CAD build for the part. Positions are in the model's coordinates, mm. A direction names the side the tool comes from. Coordinates: 2 decimals unless noted, no trailing zeros. Write each loop counter-clockwise with the first axis right and the second up, starting at its lowest first coordinate (ties: lowest second). Pieces come first, ordered by that corner, then holes. Notation, with made-up numbers: (45, -32) - (83, -32) arc R8 cw to (83, -17) - close; hole circle Ø1 at (47, -10.5). An arc over 180 degrees is marked (long way). Answer in a Markdown table with one row per item. Add a question column.
Q1. Band-saw the part on B-B (x = 0). List the corners of the cut face in (y, z).
Q2. Two-plate mould, pull along Y, no slides. Class faces 1 (the flat face through (3, -5, 115.824)), 2 (the cylindrical face through (-4.434, -3.4, 120.582)), 3 (the flat face through (0, 0, 11.176)), 4 (the cylindrical face through (0.06, 0.09, -4.32)): +Y half, -Y half, draft (parallel to the pull), parting line (faces both ways), or undercut.
Q3. 3-axis set-ups, long thin cutter, end or side, ignore diameter. For faces 5 (the flat face through (-3.937, 0, -4)), 6 (the flat face through (0, -5.588, -6)), 7 (the cylindrical face through (-1.915, -1.468, 69.126)), 8 (the flat face through (0, 5.588, -6)), 9 (the flat face through (3.937, 0, -4)): which of +Z, -Z, +X, -X, +Y, -Y reach the whole face in a straight line?
Q4. Drill centre lines: line 1 along Y through (x, z) = (0, 51); line 2 along X through (y, z) = (0.25, 56); line 3 along Y through (x, z) = (-1.5, -6.35). Where is each one in solid material? Low to high. Write a range as from..to.
Q5. Pin check, flat tips, straight feed: pin 1 (3.5 mm diameter, centred on y = 1, z = -5, fed in from -X); pin 2 (4 mm diameter, centred on x = 1, z = -3.5, fed in from -Y); pin 3 (4 mm diameter, centred on x = -1, y = 1, fed in from +Z); pin 4 (2.5 mm diameter, centred on x = 0, y = 1, fed in from +Z). Stop position of each tip, or through.
Q6. Band-saw the part on A-A (y = 0). List the corners of the cut face in (x, z), and give its area (3 significant figures).
Q7. Band-saw the part on D-D (z = 106). List the corners of the cut face in (x, y), and give its area (3 significant figures).
Q8. Band-saw the part on C-C (z = -6.35). List the corners of the cut face in (x, y).
```python
from build123d import *

# Parameters (mm, degrees)
SKETCH1_R           = 7.874
BOSS_EXTRUDE1_DEPTH = 115.824
SKETCH2_R           = 5.588
BOSS_EXTRUDE2_DEPTH = 9.652
SKETCH3_W           = 7.874
SKETCH3_H           = 11.176
BOSS_EXTRUDE3_DEPTH = 11.176
SKETCH4_R           = 2.032
CUT_EXTRUDE1_DEPTH  = 12.811
SKETCH5_R           = 2.413
CUT_EXTRUDE2_DEPTH  = 114.3


with BuildPart() as part:
    # Sketch1 → Boss-Extrude1 (new body)
    with BuildSketch(Plane.XY):
        Circle(SKETCH1_R)
    extrude(amount=BOSS_EXTRUDE1_DEPTH)

    # Sketch2 → Boss-Extrude2 (add)
    with BuildSketch(Plane.XY.offset(115.824)):
        Circle(SKETCH2_R)
    extrude(amount=BOSS_EXTRUDE2_DEPTH)

    # Sketch3 → Boss-Extrude3 (add)
    with BuildSketch(Plane(origin=(0, 0, 0), x_dir=(-1, 0, 0), z_dir=(0, 0, -1))):
        Rectangle(SKETCH3_W, SKETCH3_H)
    extrude(amount=BOSS_EXTRUDE3_DEPTH)

    # Sketch4 → Cut-Extrude1 (cut, through all)
    with BuildSketch(Plane(origin=(3.937, 0, 0), x_dir=(0, 0, -1), z_dir=(1, 0, 0))):
        with Locations((6.35, 0)):
            Circle(SKETCH4_R)
    extrude(amount=-CUT_EXTRUDE1_DEPTH, mode=Mode.SUBTRACT)

    # Sketch5 → Cut-Extrude2 (cut)
    with BuildSketch(Plane.XY.offset(125.476)):
        Circle(SKETCH5_R)
    extrude(amount=-CUT_EXTRUDE2_DEPTH, mode=Mode.SUBTRACT)


solid = part.part
```
Checked values:
| question | item | result |
|---|---|---|
| 1 | outline | (-7.87, 0) - (-5.59, 0) - (-5.59, -11.18) - (5.59, -11.18) - (5.59, 0) - (7.87, 0) - (7.87, 115.82) - (5.59, 115.82) - (5.59, 125.48) - (2.41, 125.48) - (2.41, 11.18) - (-2.41, 11.18) - (-2.41, 125.48) - (-5.59, 125.48) - (-5.59, 115.82) - (-7.87, 115.82) - close; hole circle Ø4.06 at (0, -6.35) |
| 2 | face 1 | draft |
| 2 | face 2 | parting line |
| 2 | face 3 | undercut |
| 2 | face 4 | undercut |
| 3 | face 5 | -Z, -X, +Y, -Y |
| 3 | face 6 | -Z, +X, -X, -Y |
| 3 | face 7 | +Z |
| 3 | face 8 | -Z, +X, -X, +Y |
| 3 | face 9 | -Z, +X, +Y, -Y |
| 4 | line 1 | y = -7.87..-2.41, 2.41..7.87 |
| 4 | line 2 | x = -7.87..-2.4, 2.4..7.87 |
| 4 | line 3 | y = -5.59..-2.03, 2.03..5.59 |
| 5 | pin 1 | stops at x = -3.94 |
| 5 | pin 2 | stops at y = -5.59 |
| 5 | pin 3 | stops at z = 125.48 |
| 5 | pin 4 | stops at z = 11.18 |
| 6 | outline | (-7.87, 0) - (-3.94, 0) - (-3.94, -4.32) - (3.94, -4.32) - (3.94, 0) - (7.87, 0) - (7.87, 115.82) - (5.59, 115.82) - (5.59, 125.48) - (2.41, 125.48) - (2.41, 11.18) - (-2.41, 11.18) - (-2.41, 125.48) - (-5.59, 125.48) - (-5.59, 115.82) - (-7.87, 115.82) - close; (-3.94, -11.18) - (3.94, -11.18) - (3.94, -8.38) - (-3.94, -8.38) - close |
| 6 | area | 1,440 mm² |
| 7 | outline | circle Ø15.75 at (0, 0); hole circle Ø4.83 at (0, 0) |
| 7 | area | 176 mm² |
| 8 | outline | (-3.94, -5.59) - (3.94, -5.59) - (3.94, -2.03) - (-3.94, -2.03) - close; (-3.94, 2.03) - (3.94, 2.03) - (3.94, 5.59) - (-3.94, 5.59) - close |
